Input: part model. Units: mm. Frame: model coordinates. A direction names the side the tool comes from. Round coordinates to 2 decimals unless told otherwise and drop trailing zeros. Order: outer loops, then holes, each group sorted by start corner. A loop starts at its lowest first (then second) coordinate and runs counter-clockwise, first axis right, second up.
Item 1: Mould query, pull axis Y, two halves, no side actions, for faces 3 (the flat face through (0, 0, 2.381)), 4 (the cylindrical face through (15.704, -6.511, 0.783)). Classes: released by +Y, released by -Y, zero draft, split by the parting line, or undercut.
Item 2: Line query: L1, parallel to X at y = -8, z = 0.75; L2, parallel to Y at x = -15, z = 0.3; L3, parallel to Y at x = 13, z = 1.9. Output: solid intervals per line, ascending.
Item 3: Reachability of faces 1 (the flat face through (6, -14, 1.588)), 2 (the flat face through (0, 0, 0)) from +Z, -Z, +X, -X, +Y, -Y: full face, straight path, thin tool, end or side. Return the list, or none.
Item 4: Cut plane A-A on x = 0. Output: boundary loops of the cut face in (y, z), then the cut area to 3 significant figures.
Item 5: Cut plane C-C on z = 1. Output: boundary loops of the cut face in (x, y), then the cut area to 3 significant figures.
```python
from build123d import *

# Parameters (mm, degrees)
F3_DEPTH = 2.38125
F4_DEPTH = 1.5875


# Not quite as in the source:
# - a fillet or chamfer that OpenCascade refuses, or shapes differently, is made with other operations: its cross-section is extruded or revolved along the edge and cut away or added


with BuildPart() as f3:
    # F2 (on Top) → F3 (new body)
    with BuildSketch(Plane.XY):
        with BuildLine():
            Line((-15, 0), (15, 0))
            ThreePointArc((15, 0), (0, 15), (-15, 0))
        make_face()
        with BuildLine():
            ThreePointArc((-15, 0), (0, -15), (15, 0))
            Line((15, 0), (-15, 0))
        make_face()
    extrude(amount=F3_DEPTH)

    # F2 (on Top) → F4 (join)
    with BuildSketch(Plane.XY):
        with BuildLine():
            Line((17, 0), (15, 0))
            ThreePointArc((15, 0), (0, -15), (-15, 0))
            Line((-15, 0), (-17, 0))
            ThreePointArc((-17, 0), (0, -17), (17, 0))
        make_face()
        with BuildLine():
            ThreePointArc((-15, 0), (0, 15), (15, 0))
            Line((15, 0), (17, 0))
            ThreePointArc((17, 0), (0, 17), (-17, 0))
            Line((-17, 0), (-15, 0))
        make_face()
    extrude(amount=F4_DEPTH)

    # F5: fillet of radius 0.7971733183 on 1 edges, made by hand


with BuildPart() as f5_tool2:
    # F5_s3 → F5_t4 (revolve)
    with BuildSketch(Plane.XZ):
        with BuildLine():
            ThreePointArc((-15, 1.5840766817), (-14.7665133409, 2.1477633409), (-14.2028266817, 2.38125))
            Line((-14.2028266817, 2.38125), (-15, 2.38125))
            Line((-15, 2.38125), (-15, 1.5840766817))
        make_face()
    revolve(axis=Axis((0, 0, 2.38125), (0, 0, 1)))

    split(bisect_by=Plane.XY.offset(1.5875), keep=Keep.TOP)


with BuildPart() as f3_1:
    add(f3.part)

    # F5_t1: cut F5_tool2
    add(f5_tool2.part, mode=Mode.SUBTRACT)


solid = f3_1.part
```
From the geometry:
1. face 3: zero draft
1. face 4: split by the parting line
2. L1: x = -15 to 15
2. L2: y = -8 to 8
2. L3: y = -7.35 to 7.35
3. face 1: +Z
3. face 2: -Z, +X, -X, +Y, -Y
4. outline: (-17, 0) - (17, 0) - (17, 1.59) - (15, 1.59) arc R0.8 ccw to (14.2, 2.38) - (-14.2, 2.38) arc R0.8 ccw to (-15, 1.59) - (-17, 1.59) - close
4. area: 77.5 mm2
5. outline: circle Ø34 at (0, 0)
5. area: 908 mm2
